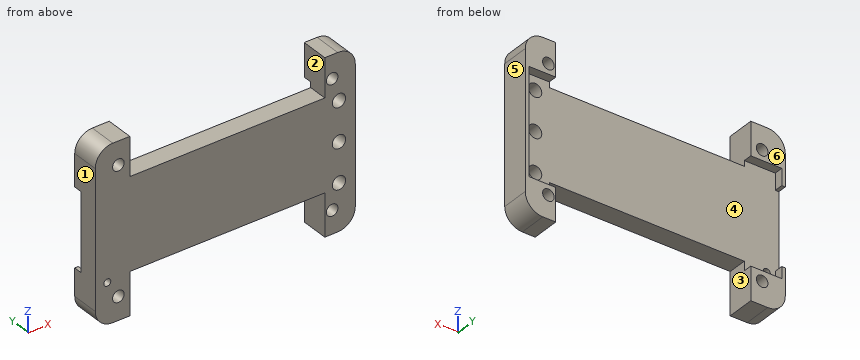
```python
from build123d import *

# Parameters (mm, degrees)
SKETCH1_W           = 74
SKETCH1_H           = 49
BOSS_EXTRUDE1_DEPTH = 7.9
FILLET1_R           = 5
SKETCH3_R           = 1.65
CUT_EXTRUDE6_DEPTH  = 7.9
SKETCH9_R           = 1.9
SKETCH9_R_2         = 1
CUT_EXTRUDE7_DEPTH  = 7.9
CUT_EXTRUDE8_DEPTH  = 2.5
SKETCH11_W          = 55.5
SKETCH11_H          = 12.1
CUT_EXTRUDE9_DEPTH  = 7.9
CUT_EXTRUDE10_DEPTH = 7.9
SKETCH15_W          = 55.5
SKETCH15_H          = 3
CUT_EXTRUDE11_DEPTH = 10


with BuildPart() as part:
    # Sketch1 → Boss-Extrude1 (new body)
    with BuildSketch(Plane(origin=(0, 0, 0), x_dir=(1, 0, 0), z_dir=(0, 1, 0))):
        Rectangle(SKETCH1_W, SKETCH1_H)
    extrude(amount=BOSS_EXTRUDE1_DEPTH)

    # Fillet1
    fillet1_edges = [part.edges().sort_by_distance(p)[0] for p in [
        (37, 3.95, 24.5),
        (-37, 3.95, 24.5),
        (-37, 3.95, -24.5),
        (37, 3.95, -24.5),
    ]]
    fillet(fillet1_edges, radius=FILLET1_R)

    # Sketch3 → Cut-Extrude6 (cut)
    with BuildSketch(Plane(origin=(0, 7.9, 0), x_dir=(1, 0, 0), z_dir=(0, 1, 0))):
        with Locations((-30.424, 17.9375)):
            Circle(SKETCH3_R)
        with Locations((30.424, 17.9375)):
            Circle(SKETCH3_R)
        with Locations((-30.424, -17.9375)):
            Circle(SKETCH3_R)
        with Locations((30.424, -17.9375)):
            Circle(SKETCH3_R)
    extrude(amount=-CUT_EXTRUDE6_DEPTH, mode=Mode.SUBTRACT)

    # Sketch9 → Cut-Extrude7 (cut)
    with BuildSketch(Plane(origin=(0, 7.9, 0), x_dir=(1, 0, 0), z_dir=(0, 1, 0))):
        with Locations((32.354, 11.2275)):
            Circle(SKETCH9_R)
        with Locations((32.354, 0.0025)):
            Circle(SKETCH9_R)
        with Locations((32.354, -11.2275)):
            Circle(SKETCH9_R)
        with Locations((-33.584, 12.9375)):
            Circle(SKETCH9_R_2)
    extrude(amount=-CUT_EXTRUDE7_DEPTH, mode=Mode.SUBTRACT)

    # Sketch10 → Cut-Extrude8 (cut)
    with BuildSketch(Plane(origin=(0, 7.9, 0), x_dir=(1, 0, 0), z_dir=(0, 1, 0))):
        Polygon((36, 15.05), (36, -15.05), (-36, -15.05), (-36, -10.35), (-37, -10.35), (-37, 11.75), (-36, 11.75), (-36, 15.05), align=None)
    extrude(amount=-CUT_EXTRUDE8_DEPTH, mode=Mode.SUBTRACT)

    # Sketch11 → Cut-Extrude9 (cut)
    with BuildSketch(Plane(origin=(0, 7.9, 0), x_dir=(1, 0, 0), z_dir=(0, 1, 0))):
        with Locations((0.574, 18.45)):
            Rectangle(SKETCH11_W, SKETCH11_H)
    extrude(amount=-CUT_EXTRUDE9_DEPTH, mode=Mode.SUBTRACT)

    # Sketch12 → Cut-Extrude10 (cut)
    with BuildSketch(Plane(origin=(0, 7.9, 0), x_dir=(1, 0, 0), z_dir=(0, 1, 0))):
        Polygon((-27.176, -15.05), (-27.176, -13.5), (28.324, -13.5), (28.324, -15.05), (28.324, -21.5), (-27.176, -21.5), align=None)
    extrude(amount=-CUT_EXTRUDE10_DEPTH, mode=Mode.SUBTRACT)

    # Sketch15 → Cut-Extrude11 (cut)
    with BuildSketch(Plane(origin=(0, 7.9, 0), x_dir=(1, 0, 0), z_dir=(0, 1, 0))):
        with Locations((0.574, -23)):
            Rectangle(SKETCH15_W, SKETCH15_H)
    extrude(amount=-CUT_EXTRUDE11_DEPTH, mode=Mode.SUBTRACT)


solid = part.part
```
Could you check a few things on this model? Use its own coordinates, in mm. Face numbers are marked on the shaded views. A direction names the side the tool comes from. Round coordinates to 2 decimals unless told otherwise and drop trailing zeros. Loops run counter-clockwise (first coordinate to the right, second up) from the corner with the lowest first, then second, coordinate; pieces in that order, holes last.
Q1. For P1, Ø2.5, axis at x = 11, y = 3.5, coming from the -Z side; P2, Ø8, axis at x = 20, z = 14, coming from the +Y side; P3, Ø1.1, axis at x = -36.5, y = 6, coming from the +Z side, each with a flat end and sliding along its axis, tell me the tip position at first contact or that it passes through.
Q2. Please list where these lines run through material, in increasing order: L1, parallel to Z at x = -30.5, y = 3; L2, parallel to X at y = 1, z = 18; L3, parallel to X at y = 7.25, z = 14.
Q3. Thinking about a two-plate mould opening in X: for the marked faces 4, 5 and 6, which applies, pulls with the +X half, pulls with the -X half, needs draft (parallel to the pull), parting line crosses it, or undercut?
Q4. I want a section at C-C (z = -20.5). Write out the boundary of the cut face in (x, y), and give its area (3 significant figures).
Q5. On a 3-axis mill with a long thin cutter (end or side, diameter ignored), from which of +Z, -Z, +X, -X, +Y, -Y can I reach the whole of each face in a straight line? I mean the marked faces 1, 2 and 3. Say none if no direction works.
Q6. I want a section at D-D (x = 17.5). Write out the boundary of the cut face in (y, z).
Q7. I want a section at A-A (y = 6.25). Write out the boundary of the cut face in (x, z), and give its area (3 significant figures).
Q8. I want a section at B-B (z = 3). Write out the boundary of the cut face in (x, y), and give its area (3 significant figures).
Answer below:
1. P1: stops at z = -12.4
1. P2: stops at y = 5.4
1. P3: stops at z = 22.57
2. L1: z = -24.5 to -19.59, -16.29 to 16.29, 19.59 to 24.5
2. L2: x = -37 to -32.07, -28.78 to -27.18, 28.32 to 28.78, 32.07 to 37
2. L3: x = -37 to -36, 36 to 37
3. face 4: undercut
3. face 5: pulls with the +X half
3. face 6: needs draft
4. outline: (-36.9, 0) - (-27.18, 0) - (-27.18, 7.9) - (-36.9, 7.9) - close; (28.32, 0) - (36.9, 0) - (36.9, 7.9) - (28.32, 7.9) - close
4. area: 145 mm2
5. face 1: +Z, -Z, -X, +Y, -Y
5. face 2: +Z, +Y, -Y
5. face 3: -Z, +Y, -Y
6. outline: (0, -12.4) - (5.4, -12.4) - (5.4, 13.5) - (0, 13.5) - close
7. outline: (-37, -19.5) arc R5 ccw to (-32, -24.5) - (-27.18, -24.5) - (-27.18, -15.05) - (-36, -15.05) - (-36, -11.75) - (-37, -11.75) - close; (-37, 10.35) - (-36, 10.35) - (-36, 15.05) - (-27.18, 15.05) - (-27.18, 24.5) - (-32, 24.5) arc R5 ccw to (-37, 19.5) - close; (28.32, -24.5) - (32, -24.5) arc R5 ccw to (37, -19.5) - (37, 19.5) arc R5 ccw to (32, 24.5) - (28.32, 24.5) - (28.32, 15.05) - (36, 15.05) - (36, -15.05) - (28.32, -15.05) - close; hole circle Ø3.3 at (-30.42, -17.94); hole circle Ø3.3 at (-30.42, 17.94); hole circle Ø3.3 at (30.42, -17.94); hole circle Ø3.3 at (30.42, 17.94)
7. area: 332 mm2
8. outline: (-37, 0) - (37, 0) - (37, 7.9) - (36, 7.9) - (36, 5.4) - (-37, 5.4) - close
8. area: 402 mm2
